Here's the drawing with two shaded views (mm, measured from the low corner). I have some questions. Coordinates: 2 decimals unless noted, no trailing zeros. Order: outer loops, then holes, each group sorted by start corner. A loop starts at its lowest first (then second) coordinate and runs counter-clockwise, first axis right, second up. Notation, with made-up numbers: M -5,48 L 38,48 A12 cw 38,52 Z; hole C 89.5,3.5 d9. An arc over 180 degrees is marked long. Put each result on its own line as item: value. Start each with the question number.
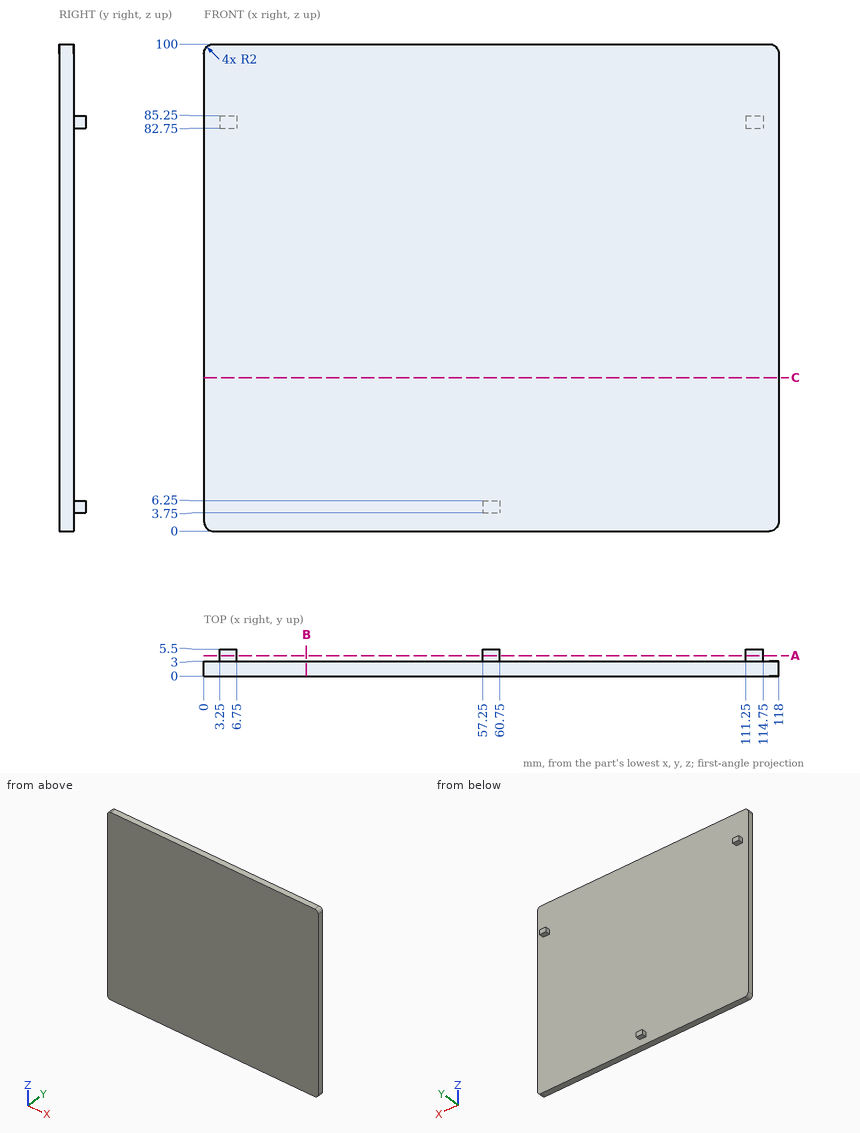
Item 1: I need wall thicknesses on probe 1 along Y at (x, z) = (105, 8.5); probe 2 along Z at (x, y) = (112.5, 4.5). Which ranges of each line are inside material? Lowest first, please.
Item 2: If we section it at A-A on y = 4.2: Write out the boundary of the cut face in (x, z).
Item 3: For pin 1 Ø0.8 at (x, y) = (112, 3.5) entering from +Z; pin 2 Ø1.2 at (x, y) = (113, 4.5) entering from -Z; pin 3 Ø0.8 at (y, z) = (4, 84.5) entering from -X; pin 4 Ø6 at (x, z) = (83, 32.5) entering from -Y, each with a flat end and sliding along its axis, tell me the tip position at first contact or that it passes through.
Item 4: If we section it at C-C on z = 31.5: Write out the boundary of the cut face in (x, y), then the cut area to 3 significant figures.
Item 5: If we section it at B-B on x = 21: Write out the boundary of the cut face in (y, z), then the cut area to 3 significant figures.
Geometry check:
1. probe 1: y = 0 to 3
1. probe 2: z = 82.75 to 85.25
2. outline: M 3.25,82.75 L 6.75,82.75 L 6.75,85.25 L 3.25,85.25 Z; M 57.25,3.75 L 60.75,3.75 L 60.75,6.25 L 57.25,6.25 Z; M 111.25,82.75 L 114.75,82.75 L 114.75,85.25 L 111.25,85.25 Z
3. pin 1: stops at z = 85.25
3. pin 2: stops at z = 82.75
3. pin 3: stops at x = 3.25
3. pin 4: stops at y = 0
4. outline: M 0,0 L 118,0 L 118,3 L 0,3 Z
4. area: 354 mm²
5. outline: M 0,0 L 3,0 L 3,100 L 0,100 Z
5. area: 300 mm²
